from build123d import *

# Parameters (mm, degrees)
SKETCH_1_W             = 150
SKETCH_1_H             = 36
EXTRUDE_2_DEPTH        = 6
SKETCH_6_W             = 10
SKETCH_6_H             = 6
EXTRUDE_4_DEPTH        = 4
PATTERN_LINEAR_1_COUNT = 6
PATTERN_LINEAR_1_PITCH = 25
SKETCH_8_W             = 5
SKETCH_8_H             = 6
SKETCH_8_W_2           = 4.995224333
CUT_EXTRUDE_3_DEPTH    = 6
SKETCH_11_W            = 4.504775667
SKETCH_11_H            = 6
SKETCH_11_W_2          = 4.5
CUT_EXTRUDE_4_DEPTH    = 6
SKETCH_12_W            = 35.2
SKETCH_12_H            = 25.2
CUT_EXTRUDE_5_DEPTH    = 155.376163963
SKETCH_14_W            = 15
SKETCH_14_H            = 6
SKETCH_14_W_2          = 10
CUT_EXTRUDE_6_DEPTH    = 4
SKETCH_15_W            = 15
SKETCH_15_H            = 6
EXTRUDE_5_DEPTH        = 1
PATTERN_LINEAR_2_COUNT = 5
PATTERN_LINEAR_2_PITCH = 25
SKETCH_16_W            = 15
SKETCH_16_H            = 6
EXTRUDE_6_DEPTH        = 1
SKETCH_17_W            = 10
SKETCH_17_H            = 6
EXTRUDE_7_DEPTH        = 1
SKETCH_18_W            = 15
SKETCH_18_H            = 6
EXTRUDE_8_DEPTH        = 1
SKETCH_19_W            = 6
SKETCH_19_H            = 6
EXTRUDE_9_DEPTH        = 3


with BuildPart() as part:
    # Эскиз1 → Бобышка-Вытянуть2 (new body)
    with BuildSketch(Plane(origin=(0, 0, 0), x_dir=(1, 0, 0), z_dir=(0, 1, 0))):
        with Locations((75, -18)):
            Rectangle(SKETCH_1_W, SKETCH_1_H)
    extrude(amount=EXTRUDE_2_DEPTH)

    # Эскиз6 → Бобышка-Вытянуть4 (add)
    with BuildSketch(Plane(origin=(0, 0, 0), x_dir=(-1, 0, 0), z_dir=(0, 0, -1))):
        with Locations((-5, 3)):
            Rectangle(SKETCH_6_W, SKETCH_6_H)
    extrude_4 = extrude(amount=EXTRUDE_4_DEPTH)

    # Линейный массив1: Бобышка-Вытянуть4 ×6
    with Locations(*[(i * PATTERN_LINEAR_1_PITCH, 0, 0) for i in range(1, PATTERN_LINEAR_1_COUNT)]):
        add(extrude_4)

    # Эскиз8 → Вырез-Вытянуть3 (cut)
    with BuildSketch(Plane.ZY):
        with Locations((6.5, 3)):
            Rectangle(SKETCH_8_W, SKETCH_8_H)
        with Locations((16, 3)):
            Rectangle(SKETCH_8_W, SKETCH_8_H)
        with Locations((25.502387834, 3)):
            Rectangle(SKETCH_8_W_2, SKETCH_8_H)
    extrude(amount=-CUT_EXTRUDE_3_DEPTH, mode=Mode.SUBTRACT)

    # Эскиз11 → Вырез-Вытянуть4 (cut)
    with BuildSketch(Plane(origin=(150, 0, 0), x_dir=(0, 0, -1), z_dir=(1, 0, 0))):
        with Locations((-20.752387834, 3)):
            Rectangle(SKETCH_11_W, SKETCH_11_H)
        with Locations((-11.25, 3)):
            Rectangle(SKETCH_11_W_2, SKETCH_11_H)
    extrude(amount=-CUT_EXTRUDE_4_DEPTH, mode=Mode.SUBTRACT)

    # Эскиз12 → Вырез-Вытянуть5 (cut, through all)
    with BuildSketch(Plane(origin=(0, 6, 0), x_dir=(1, 0, 0), z_dir=(0, 1, 0))):
        with Locations((67.6, -19.4)):
            Rectangle(SKETCH_12_W, SKETCH_12_H)
    extrude(amount=-CUT_EXTRUDE_5_DEPTH, mode=Mode.SUBTRACT)

    # Эскиз14 → Вырез-Вытянуть6 (cut)
    with BuildSketch(Plane.XY.offset(36)):
        with Locations((17.5, 3)):
            Rectangle(SKETCH_14_W, SKETCH_14_H)
        with Locations((130, 3)):
            Rectangle(SKETCH_14_W_2, SKETCH_14_H)
    extrude(amount=-CUT_EXTRUDE_6_DEPTH, mode=Mode.SUBTRACT)

    # Эскиз15 → Бобышка-Вытянуть5 (add)
    with BuildSketch(Plane(origin=(0, 0, 0), x_dir=(-1, 0, 0), z_dir=(0, 0, -1))):
        with Locations((-17.5, 3)):
            Rectangle(SKETCH_15_W, SKETCH_15_H)
    extrude_5 = extrude(amount=EXTRUDE_5_DEPTH)

    # Линейный массив2: Бобышка-Вытянуть5 ×5
    with Locations(*[(i * PATTERN_LINEAR_2_PITCH, 0, 0) for i in range(1, PATTERN_LINEAR_2_COUNT)]):
        add(extrude_5)

    # Эскиз16 → Бобышка-Вытянуть6 (add)
    with BuildSketch(Plane(origin=(0, 0, 0), x_dir=(-1, 0, 0), z_dir=(0, 0, -1))):
        with Locations((-142.5, 3)):
            Rectangle(SKETCH_16_W, SKETCH_16_H)
    extrude(amount=EXTRUDE_6_DEPTH)

    # Эскиз17 → Бобышка-Вытянуть7 (add)
    with BuildSketch(Plane.XY.offset(32)):
        with Locations((130, 3)):
            Rectangle(SKETCH_17_W, SKETCH_17_H)
    extrude(amount=EXTRUDE_7_DEPTH)

    # Эскиз18 → Бобышка-Вытянуть8 (add)
    with BuildSketch(Plane.XY.offset(32)):
        with Locations((17.5, 3)):
            Rectangle(SKETCH_18_W, SKETCH_18_H)
    extrude(amount=EXTRUDE_8_DEPTH)

    # Эскиз19 → Бобышка-Вытянуть9 (add)
    with BuildSketch(Plane(origin=(0, 0, -1), x_dir=(-1, 0, 0), z_dir=(0, 0, -1))):
        with Locations((-147, 3)):
            Rectangle(SKETCH_19_W, SKETCH_19_H)
    extrude(amount=EXTRUDE_9_DEPTH)


solid = part.part
Check sheet for the modelled part. Datum: model origin and axes. Units: mm. A direction names the side the tool comes from. Round coordinates to 2 decimals unless told otherwise and drop trailing zeros. Order: outer loops, then holes, each group sorted by start corner. A loop starts at its lowest first (then second) coordinate and runs counter-clockwise, first axis right, second up.
(1) Cross-section at B-B, the plane x = 64. Enter the section's corners in (y, z), and give its area (3 significant figures).
(2) Cross-section at D-D, the plane x = 42. Enter the section's corners in (y, z).
(3) Draft check along Z on faces 5 (the flat face through (17, 3, 33)), 6 (the flat face through (50, 3, 20)), 7 (the flat face through (0, 3, 32)). Enter one of: pulls with the +Z half, pulls with the -Z half, needs draft (parallel to the pull), parting line crosses it, or undercut.
(4) Cross-section at C-C, the plane x = 23. Enter the section's corners in (y, z).
(5) Scan lines: probe 1 along X at (y, z) = (4.4, 8.5); probe 2 along X at (y, z) = (4.1, 22); probe 3 along Z at (x, y) = (58, 1.2). Record each from-to range of solid material in increasing order.
(6) Go/stop test with flat-tipped pins: P1, Ø0.9, axis at y = 4, z = 34.5, coming from the -X side; P2, Ø2.5, axis at y = 3.5, z = 7.5, coming from the -X side; P3, Ø1.8, axis at x = 71, y = 3, coming from the -Z side. Record where each tip stops, or that it passes through.
(7) Cross-section at A-A, the plane z = 15. Enter the section's corners in (x, y), and give its area (3 significant figures).
(8) Access from +Z, -Z, +X, -X, +Y, -Y to the whole of each face (thin tool, end or side, straight path). Record for faces 1 (the flat face through (130, 3, 33)), 2 (the flat face through (3, 3, 23.005)), 3 (the flat face through (68, 3, -1)), 4 (the flat face through (147, 3, 13.5)).
Check sheet entries:
1. outline: (0, -1) - (6, -1) - (6, 6.8) - (0, 6.8) - close; (0, 32) - (6, 32) - (6, 36) - (0, 36) - close
1. area: 70.8 mm2
2. outline: (0, -1) - (6, -1) - (6, 36) - (0, 36) - close
3. face 5: pulls with the +Z half
3. face 6: undercut
3. face 7: needs draft
4. outline: (0, -1) - (6, -1) - (6, 33) - (0, 33) - close
5. probe 1: x = 6 to 50, 85.2 to 150
5. probe 2: x = 0 to 50, 85.2 to 144
5. probe 3: z = -4 to 6.8, 32 to 36
6. P1: stops at x = 0
6. P2: stops at x = 6
6. P3: stops at z = -1
7. outline: (6, 0) - (50, 0) - (50, 6) - (6, 6) - close; (85.2, 0) - (150, 0) - (150, 6) - (85.2, 6) - close
7. area: 653 mm2
8. face 1: +Z, +Y, -Y
8. face 2: -X, +Y, -Y
8. face 3: -Z, +Y, -Y
8. face 4: +X, +Y, -Y
